```python
from build123d import *

# Parameters (mm, degrees)
SKETCH2_R                       = 4
BOSS_EXTRUDE1_DEPTH             = 5
SKETCH3_R                       = 5.75
BOSS_EXTRUDE2_DEPTH             = 16
SKETCH4_W                       = 15
SKETCH4_H                       = 15
BOSS_EXTRUDE3_DEPTH             = 20
M2X0_4_TAPPED_HOLE1_D           = 1.6
M2X0_4_TAPPED_HOLE1_DEPTH       = 15
M2X0_4_TAPPED_HOLE1_CSINK_D     = 2.05
M2X0_4_TAPPED_HOLE1_CSINK_ANGLE = 90
M2X0_4_TAPPED_HOLE1_TIP         = 0.480688495
SKETCH10_R                      = 6.25
BOSS_EXTRUDE4_DEPTH             = 3
SKETCH11_W                      = 2
SKETCH11_H                      = 3
CUT_EXTRUDE2_DEPTH              = 5


with BuildPart() as part:
    # Sketch2 → Boss-Extrude1 (new body)
    with BuildSketch(Plane(origin=(0, 0, 0), x_dir=(1, 0, 0), z_dir=(0, 1, 0))):
        with Locations(Location((0, 0, 0), (0, 0, 270))):
            Circle(SKETCH2_R)
    extrude(amount=BOSS_EXTRUDE1_DEPTH)

    # Sketch3 → Boss-Extrude2 (add)
    with BuildSketch(Plane(origin=(0, 5, 0), x_dir=(1, 0, 0), z_dir=(0, 1, 0))):
        with Locations(Location((0, 0, 0), (0, 0, 270))):
            Circle(SKETCH3_R)
    extrude(amount=BOSS_EXTRUDE2_DEPTH)

    # Sketch4 → Boss-Extrude3 (add)
    with BuildSketch(Plane(origin=(0, 21, 0), x_dir=(1, 0, 0), z_dir=(0, 1, 0))):
        Rectangle(SKETCH4_W, SKETCH4_H)
    extrude(amount=BOSS_EXTRUDE3_DEPTH)

    # M2x0.4 Tapped Hole1
    with Locations(Plane(origin=(0, 0, 0), x_dir=(-1, 0, 0), z_dir=(0, -1, 0))):
        with Locations((0, 0)):
            CounterSinkHole(M2X0_4_TAPPED_HOLE1_D / 2, M2X0_4_TAPPED_HOLE1_CSINK_D / 2, depth=M2X0_4_TAPPED_HOLE1_DEPTH, counter_sink_angle=M2X0_4_TAPPED_HOLE1_CSINK_ANGLE)
            with Locations((0, 0, -(M2X0_4_TAPPED_HOLE1_DEPTH + M2X0_4_TAPPED_HOLE1_TIP / 2))):  # 118° drill point
                Cone(0, M2X0_4_TAPPED_HOLE1_D / 2, M2X0_4_TAPPED_HOLE1_TIP, mode=Mode.SUBTRACT)

    # Sketch10 → Boss-Extrude4 (add)
    with BuildSketch(Plane.XZ.offset(-21)):
        with Locations(Location((0, 0, 0), (0, 0, 270))):
            Circle(SKETCH10_R)
    extrude(amount=BOSS_EXTRUDE4_DEPTH)

    # Sketch11 → Cut-Extrude2 (cut)
    with BuildSketch(Plane.XZ):
        with Locations((0, 4)):
            Rectangle(SKETCH11_W, SKETCH11_H)
    extrude(amount=-CUT_EXTRUDE2_DEPTH, mode=Mode.SUBTRACT)


solid = part.part
```
Here's how the part is built. I have some questions about the finished solid (model axes, mm). A direction names the side the tool comes from. Give positions to 0.01 mm unless a question says otherwise; leave off trailing zeros. Loops run counter-clockwise (first coordinate to the right, second up) from the corner with the lowest first, then second, coordinate; pieces in that order, holes last. Notation, with made-up numbers: M -30,-24.5 L 16,-24.5 A26 cw 16,13.5 Z; hole C 10.25,-6.5 d8. An arc over 180 degrees is marked long. Put each result on its own line as item: value. Start each with the question number.
(1) I want a section at D-D on x = -3. Please give me the cut outline in (y, z), then the cut area to 3 significant figures.
(2) If we mould it in two halves opening along Z, with no side actions, what happens to faces 1 (the conical face through (0.139, 15.397, -0.006)), 2 (the flat face through (0, 31, -7.5)), 3 (the flat face through (0, 31, 7.5)), 4 (the flat face through (7.5, 31, 0))? For each: +Z half, -Z half, draft (parallel to the pull), parting line (faces both ways), or undercut.
(3) I want a section at A-A on y = 3. Please give me the cut outline in (x, z), then the cut area to 3 significant figures.
(4) I need wall thicknesses on line 1 along Z through (x, y) = (0, 11); line 2 along Y through (x, z) = (-4, 1); line 3 along Y through (x, z) = (-5.25, 6.5). Which ranges of each line are inside material? Lowest first, please. Write a range as [from, to].
(5) I want a section at C-C on z = 4.5. Please give me the cut outline in (x, y), then the cut area to 3 significant figures.
(6) For faces 5 (the flat face through (-7, 21, 0)), 6 (the flat face through (0, 2, 2.5)), 7 (the flat face through (0, 41, 0)), which set-ups out of +Z, -Z, +X, -X, +Y, -Y let a thin tool reach every point of the face, with its end or its side?
(7) Will these pins go through, and if not, where does the flat tip stop? pin 1 Ø2 at (x, y) = (-4.5, 14.5) entering from -Z; pin 2 Ø1 at (x, y) = (0, 3) entering from +Z; pin 3 Ø1 at (x, z) = (3, -0.5) entering from -Y; pin 4 Ø1 at (x, z) = (-5, -3.5) entering from -Y.
(8) I want a section at B-B on x = 2.25. Please give me the cut outline in (y, z).
Answer block:
1. outline: M 0,-2.65 L 5,-2.65 L 5,-4.91 L 18,-4.91 L 18,-5.48 L 21,-5.48 L 21,-7.5 L 41,-7.5 L 41,7.5 L 21,7.5 L 21,5.48 L 18,5.48 L 18,4.91 L 5,4.91 L 5,2.65 L 0,2.65 Z
1. area: 487 mm^2
2. face 1: undercut
2. face 2: -Z half
2. face 3: +Z half
2. face 4: draft
3. outline: M -1,2.5 L -1,3.87 A4 ccw long 1,3.87 L 1,2.5 Z; hole C 0,0 d1.6
3. area: 45.3 mm^2
4. line 1: [-5.75, -0.8], [0.8, 5.75]
4. line 2: [5, 41]
4. line 3: [21, 41]
5. outline: M -7.5,21 L -4.34,21 L -4.34,18 L -3.58,18 L -3.58,5 L 3.58,5 L 3.58,18 L 4.34,18 L 4.34,21 L 7.5,21 L 7.5,41 L -7.5,41 Z
5. area: 419 mm^2
6. face 5: -Y
6. face 6: +Z, -Y
6. face 7: +Z, -Z, +X, -X, +Y
7. pin 1: z = -4.56
7. pin 2: z = 2.5
7. pin 3: y = 0
7. pin 4: y = 5
8. outline: M 0,-3.31 L 5,-3.31 L 5,-5.29 L 18,-5.29 L 18,-5.83 L 21,-5.83 L 21,-7.5 L 41,-7.5 L 41,7.5 L 21,7.5 L 21,5.83 L 18,5.83 L 18,5.29 L 5,5.29 L 5,3.31 L 0,3.31 Z
